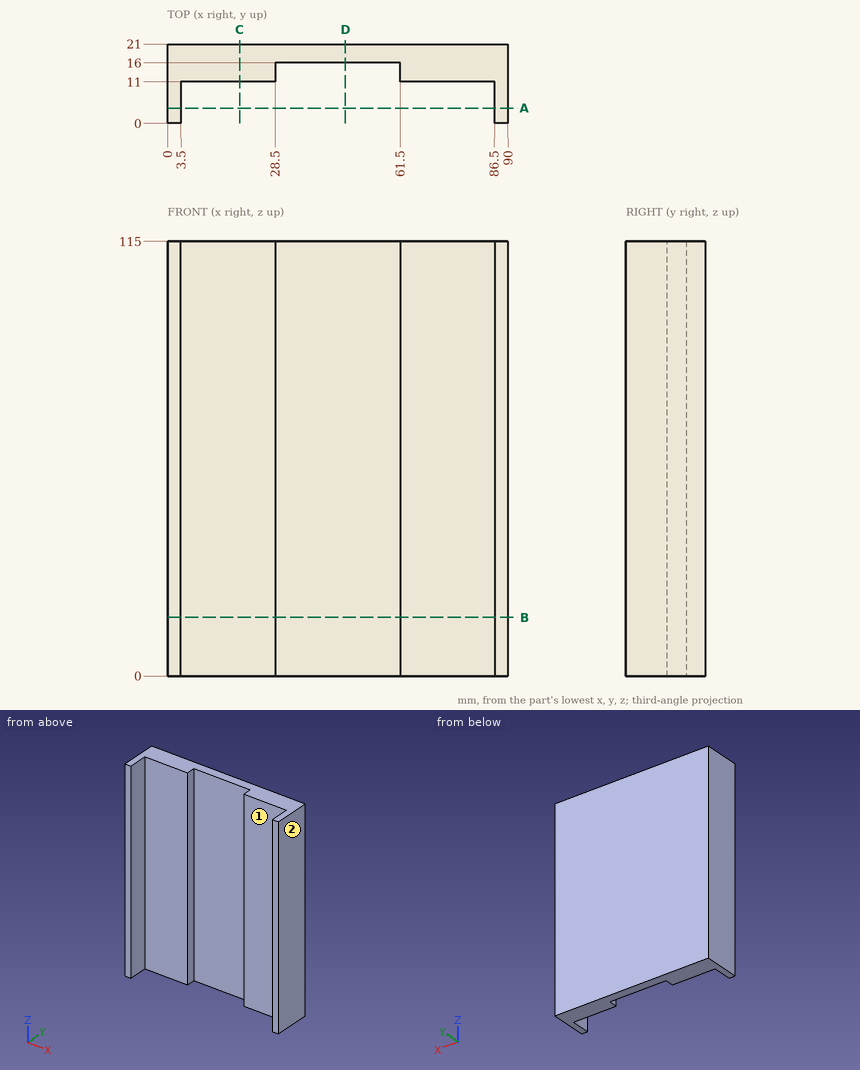
The drawing under review shows one solid part. Ordinate dimensions are in mm from its lowest x, y, z. A direction names the side the tool comes from. Give positions to 0.01 mm unless a question says otherwise; leave off trailing zeros. Order: outer loops, then holes, each group sorted by start corner. A loop starts at its lowest first (then second) coordinate and runs counter-clockwise, first axis right, second up. Notation, with made-up numbers: (51.25, 76.25) -> (72.25, 76.25) arc R33 ccw to (72.25, 109.25) -> close; hole circle Ø3 at (78, 89). An arc over 180 degrees is marked (long way). Write item = value, one per line.
1) Insertion check: pin 1 (12.5 mm diameter, centred on x = 78, z = 29, fed in from -Y); pin 2 (4 mm diameter, centred on x = 49, z = 28, fed in from -Y); pin 3 (2 mm diameter, centred on x = 69.5, y = 17, fed in from -Z). Each pin has a flat end and moves straight along its axis. Give the tip position at first contact, or say it passes through.
Findings:
pin_1 = 11
pin_2 = 16
pin_3 = 0
2) We need section C-C, the plane x = 19. Give the boundary of the cut face in (y, z), and give its area (3 significant figures).
Findings:
outline = (11, 0) -> (21, 0) -> (21, 115) -> (11, 115) -> close
area = 1,150 mm^2
3) For the marked faces 1 and 2, list the 3-axis set-ups (+Z, -Z, +X, -X, +Y, -Y) from which the entire face can be reached by the end or side of a thin tool; tool diameter is ignored.
Findings:
face_1 = +Z, -Z, -Y
face_2 = +Z, -Z, +X, +Y, -Y
4) We need section D-D, the plane x = 47. Give the boundary of the cut face in (y, z), and give its area (3 significant figures).
Findings:
outline = (16, 0) -> (21, 0) -> (21, 115) -> (16, 115) -> close
area = 575 mm^2
5) We need section B-B, the plane z = 15.5. Give the boundary of the cut face in (x, y), and give its area (3 significant figures).
Findings:
outline = (0, 0) -> (3.5, 0) -> (3.5, 11) -> (28.5, 11) -> (28.5, 16) -> (61.5, 16) -> (61.5, 11) -> (86.5, 11) -> (86.5, 0) -> (90, 0) -> (90, 21) -> (0, 21) -> close
area = 812 mm^2
6) To check wall thickness, follow L1, parallel to X at y = 11.75, z = 27; L2, parallel to X at y = 2.75, z = 53; L3, parallel to Y at x = 67.5, z = 5. State the ranges of each line that lie inside material, in increasing order. Write a range as from..to.
Findings:
L1 = 0..28.5, 61.5..90
L2 = 0..3.5, 86.5..90
L3 = 11..21
7) We need section A-A, the plane y = 4. Give the boundary of the cut face in (x, z).
Findings:
outline = (0, 0) -> (3.5, 0) -> (3.5, 115) -> (0, 115) -> close; (86.5, 0) -> (90, 0) -> (90, 115) -> (86.5, 115) -> close
